Check sheet for the modelled part. Datum: model origin and axes. Units: mm. A direction names the side the tool comes from. Coordinates: 2 decimals unless noted, no trailing zeros. Loops run counter-clockwise (first coordinate to the right, second up) from the corner with the lowest first, then second, coordinate; pieces in that order, holes last. Notation, with made-up numbers: M 30,-1.5 L 44,-1.5 A15 ccw 44,27.5 Z; hole C -4.75,23 d5. An arc over 180 degrees is marked long. Answer as CSV lines item,"result". Start each with the question number.
from build123d import *

# Parameters (mm, degrees)
SALIENTE_EXTRUIR2_DEPTH    = 30
CROQUIS3_W                 = 60.629420227
CROQUIS3_H                 = 60.965705304
CORTAR_EXTRUIR1_DEPTH      = 30
CROQUIS4_R                 = 3
CORTAR_EXTRUIR2_DEPTH      = 88.482529848
CROQUIS5_W                 = 28.284271248
CROQUIS5_H                 = 30
SALIENTE_EXTRUIR3_DEPTH    = 14.142136
SALIENTE_EXTRUIR4_DEPTH    = 10
CROQUIS7_W                 = 23.581736244
CROQUIS7_H                 = 30.206171788
CORTAR_EXTRUIR3_DEPTH      = 60
CROQUIS8_R                 = 3
CORTAR_EXTRUIR4_DEPTH      = 99.7393004
CROQUIS10_W                = 79.072347139
CROQUIS10_H                = 56.401254602
CORTAR_EXTRUIR5_DEPTH      = 50
CORTAR_EXTRUIR6_DEPTH      = 66
CORTAR_EXTRUIR6_DEPTH_BACK = 97
CROQUIS11_W                = 135.934764717
CROQUIS11_H                = 98.230231438


with BuildPart() as part:
    # Croquis2 → Saliente-Extruir2 (new body)
    with BuildSketch(Plane(origin=(0, 0, 0), x_dir=(0, 0, -1), z_dir=(1, 0, 0))):
        Polygon((0, 0), (-50, 0), (-75.724787771, -15.434872663), (-75.724787771, -45.434872663), (-55.724787771, -45.434872663), (-55.724787771, -26.758680242), (-44.460320701, -20), (0, -20), align=None)
    extrude(amount=SALIENTE_EXTRUIR2_DEPTH)

    # Croquis3 → Cortar-Extruir1 (cut)
    with BuildSketch(Plane(origin=(-22.862393886, 0, 22.862393886), x_dir=(0.7071067811865462, 0, 0.7071067811865488), z_dir=(-0.7071067811865488, 0, 0.7071067811865462))):
        with Locations((51.516510193, -19.86952732)):
            Rectangle(CROQUIS3_W, CROQUIS3_H)
    extrude(amount=CORTAR_EXTRUIR1_DEPTH, mode=Mode.SUBTRACT)

    # Croquis4 → Cortar-Extruir2 (cut, through all)
    with BuildSketch(Plane(origin=(-22.862393886, 0, 22.862393886), x_dir=(0.7071067811865461, 0, 0.7071067811865489), z_dir=(-0.7071067811865489, 0, 0.7071067811865461))):
        with Locations((60.616578749, -34.226076292)):
            Circle(CROQUIS4_R)
    extrude(amount=-CORTAR_EXTRUIR2_DEPTH, mode=Mode.SUBTRACT)

    # Croquis5 → Saliente-Extruir3 (add)
    with BuildSketch(Plane(origin=(-22.862393886, 0, 22.862393886), x_dir=(0.7071067811865461, 0, 0.7071067811865489), z_dir=(-0.7071067811865489, 0, 0.7071067811865461))):
        with Locations((60.616578749, -30.434872663)):
            Rectangle(CROQUIS5_W, CROQUIS5_H)
    extrude(amount=-SALIENTE_EXTRUIR3_DEPTH)

    # Croquis6 → Saliente-Extruir4 (add)
    with BuildSketch(Plane(origin=(-22.862393886, 0, 22.862393886), x_dir=(0.7071067811865461, 0, 0.7071067811865489), z_dir=(-0.7071067811865489, 0, 0.7071067811865461))):
        Polygon((32.332307501, -20.758680242), (46.474443125, -26.758680242), (46.474443125, -45.434872663), (74.758714373, -45.434872663), (74.758714373, -15.434872663), (38.378370617, 0), (32.332307501, 0), align=None)
    extrude(amount=SALIENTE_EXTRUIR4_DEPTH)

    # Croquis7 → Cortar-Extruir3 (cut)
    with BuildSketch(Plane(origin=(0, 0, 0), x_dir=(1, 0, 0), z_dir=(0, 1, 0))):
        with Locations((-11.790868122, -58.05803285)):
            Rectangle(CROQUIS7_W, CROQUIS7_H)
    extrude(amount=-CORTAR_EXTRUIR3_DEPTH, mode=Mode.SUBTRACT)

    # Croquis8 → Cortar-Extruir4 (cut, through all)
    with BuildSketch(Plane(origin=(-29.933461698, 0, 29.933461698), x_dir=(0.707106781186546, 0, 0.7071067811865491), z_dir=(-0.7071067811865491, 0, 0.707106781186546))):
        with Locations((60.616578749, -35.434872663)):
            Circle(CROQUIS8_R)
    extrude(amount=-CORTAR_EXTRUIR4_DEPTH, mode=Mode.SUBTRACT)

    # Croquis10 → Cortar-Extruir5 (cut)
    with BuildSketch(Plane(origin=(0, 22.058823529, 13.235294118), x_dir=(1, 0, 0), z_dir=(0, 0.8574929257125444, 0.5144957554275262))):
        with Locations((7.523719949, -68.590647859)):
            Rectangle(CROQUIS10_W, CROQUIS10_H)
    extrude(amount=CORTAR_EXTRUIR5_DEPTH, mode=Mode.SUBTRACT)


with BuildPart() as body_2:
    # Simetría3: mirrored copy
    add(part.part.mirror(Plane(origin=(0, 0, -5), x_dir=(1, 0, 0), z_dir=(0, 0, -1))))


with BuildPart() as part_1:
    add(part.part)

    # Croquis11 → Cortar-Extruir6 (cut, two sides: drawn at the far end of the back side and taken through both)
    with BuildSketch(Plane.XZ.offset(20).offset(-CORTAR_EXTRUIR6_DEPTH_BACK)):
        with Locations((20.973016289, 43.122891159)):
            Rectangle(CROQUIS11_W, CROQUIS11_H)
    extrude(amount=CORTAR_EXTRUIR6_DEPTH + CORTAR_EXTRUIR6_DEPTH_BACK, mode=Mode.SUBTRACT)


solid = body_2.part
Item 1: Set-up check for faces 1 (the face through (14.79, -21.925, -57.668)), 2 (the face through (29.86, -30.225, -65.585)), 3 (the face through (15, -20, -33)), 4 (the face through (11.584, -35.666, -64.141)), 5 (the face through (21, -45.435, -74)): record each of +Z, -Z, +X, -X, +Y, -Y from which the full face is reachable in a straight line by a thin tool's end or side.
Item 2: Sectioned sample at D-D, the plane y = -23. Record the boundary of the cut face in (x, z).
Item 3: Go/stop test with flat-tipped pins: pin 1 (12 mm diameter, centred on x = 34, y = -19, fed in from -Z); pin 2 (1.5 mm diameter, centred on x = 25.5, z = -82.5, fed in from +Y); pin 3 (3 mm diameter, centred on x = 15, z = -65, fed in from +Y); pin 4 (12 mm diameter, centred on x = 29, z = -58, fed in from -Y). Record where each tip stops, or that it passes through.
Item 4: Material ranges on line 1 (Y direction, x = 6, z = -44); line 2 (X direction, y = -21.5, z = -60); line 3 (X direction, y = -36, z = -78.5), recorded low to high. Write a range as from..to.
Item 5: Sectioned sample at C-C, the plane x = 7.5. Record the boundary of the cut face in (y, z).
Item 6: Sectioned sample at B-B, the plane z = -24. Record the boundary of the cut face in (x, y), and give its area (3 significant figures).
Item 7: Sectioned sample at A-A, the plane y = -18. Record the boundary of the cut face in (x, z).
Item 8: Release check for a two-part mould opening along Y. For faces 6 (the face through (0, -10, -40)), 7 (the face through (34, -15.435, -76)), 8 (the face through (20.885, -38.364, -73.92)) record: released by +Y, released by -Y, zero draft, split by the parting line, or undercut.
Reply:
1,face 1,"+Z, -Y"
1,face 2,"+Z, +X, -Y"
1,face 3,"+Z, +X, -X, -Y"
1,face 4,"+Z, -X, -Y"
1,face 5,"+Z, -Z, +X, -X, -Y"
2,outline,"M 0,-69.87 L 22.93,-92.8 L 40,-75.72 L 30,-65.72 L 30,-59.46 L 23.74,-59.46 L 20,-55.72 L 16.26,-59.46 L 3.74,-59.46 L 0,-63.2 Z"
3,pin 1,"z = -87.72"
3,pin 2,"y = -13.05"
3,pin 3,"y = -2.1"
3,pin 4,"y = -45.43"
4,line 1,"-20..0"
4,line 2,"0..30"
4,line 3,"8.63..13.06, 21.39..37.22"
5,outline,"M -45.43,-77.37 L -10.42,-77.37 L 0,-60 L 0,-10 L -20,-10 L -20,-54.46 L -25.26,-63.22 L -26.76,-68.22 L -45.43,-68.22 Z"
6,outline,"M 0,-20 L 30,-20 L 30,0 L 0,0 Z"
6,area,"600 mm²"
7,outline,"M 0,-69.87 L 20.13,-90 L 25.72,-90 L 40,-75.72 L 30,-65.72 L 30,-10 L 0,-10 Z"
8,face 6,"zero draft"
8,face 7,"released by +Y"
8,face 8,"undercut"
